```python
from build123d import *

# Parameters (mm, degrees)
F0_R     = 19.2
F1_DEPTH = 20
F2_R     = 2
F3_DEPTH = 25


with BuildPart() as f1:
    # F0 (on Top) → F1 (new body)
    with BuildSketch(Plane.XY):
        with BuildLine():
            ThreePointArc((14.459278, -13.962065), (18.636543, -7.529227), (20.1, 0))
            ThreePointArc((20.1, 0), (-7.529227, 18.636543), (-14.459278, -13.962065))
            ThreePointArc((-14.459278, -13.962065), (-7.854059, -18.501993), (0, -20.1))
            ThreePointArc((0, -20.1), (7.854059, -18.501993), (14.459278, -13.962065))
        make_face()
        Circle(F0_R, mode=Mode.SUBTRACT)
        Polygon((0, -23.1), (0, -20.1), (-20.239076, -20.1), (-30, -20.1), (-30, -23.1), align=None)
        with BuildLine():
            Line((20.239076, -20.1), (14.459278, -13.962065))
            ThreePointArc((14.459278, -13.962065), (7.854059, -18.501993), (0, -20.1))
            Line((0, -20.1), (20.239076, -20.1))
        make_face()
        with BuildLine():
            ThreePointArc((0, -20.1), (-7.854059, -18.501993), (-14.459278, -13.962065))
            Line((-14.459278, -13.962065), (-20.239076, -20.1))
            Line((-20.239076, -20.1), (0, -20.1))
        make_face()
        Polygon((20.239076, -20.1), (0, -20.1), (0, -23.1), (30, -23.1), (30, -20.1), align=None)
    extrude(amount=F1_DEPTH)

    # F2 (on face) → F3 (cut)
    with BuildSketch(Plane(origin=(0, -20.1, 0), x_dir=(-1, 0, 0), z_dir=(0, 1, 0))):
        with BuildLine():
            Line((-25.119538, 10.263338), (-25.119538, 8.263338))
            ThreePointArc((-25.119538, 8.263338), (-23.705324, 8.849124), (-23.119538, 10.263338))
            ThreePointArc((-23.119538, 10.263338), (-25.119538, 12.263338), (-27.119538, 10.263338))
            Line((-27.119538, 10.263338), (-25.119538, 10.263338))
        make_face()
        with BuildLine():
            ThreePointArc((-27.119538, 10.263338), (-26.533751, 8.849124), (-25.119538, 8.263338))
            Line((-25.119538, 8.263338), (-25.119538, 10.263338))
            Line((-25.119538, 10.263338), (-27.119538, 10.263338))
        make_face()
        with Locations((25.119538, 10.263338)):
            Circle(F2_R)
    extrude(amount=-F3_DEPTH, mode=Mode.SUBTRACT)


solid = f1.part
```
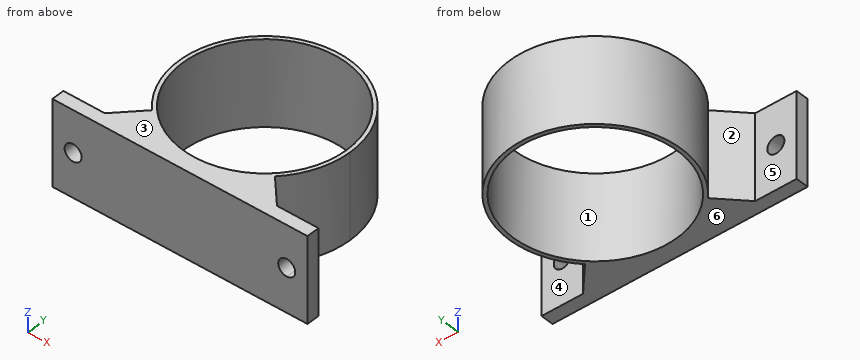
Could you check a few things on this model? Use its own coordinates, in mm. Face numbers are marked on the shaded views. A direction names the side the tool comes from. Round coordinates to 2 decimals unless told otherwise and drop trailing zeros. Loops run counter-clockwise (first coordinate to the right, second up) from the corner with the lowest first, then second, coordinate; pieces in that order, holes last. Notation, with made-up numbers: (52, -26.5) - (101, -26.5) arc R21 ccw to (101, -2.5) - close; hole circle Ø5 at (-10.75, -19.75). An arc over 180 degrees is marked (long way). Answer in a Markdown table with one row per item. Add a question column.
(1) For the marked faces 4, 5 and 6, which set-ups out of +Z, -Z, +X, -X, +Y, -Y let a thin tool reach every point of the face, with its end or its side?
(2) I'm going to push flat-ended pins straight in: pin 1 (3 mm diameter, centred on y = 12, z = 14, fed in from +X); pin 2 (6 mm diameter, centred on y = -14.5, z = 2.5, fed in from -X); pin 3 (8 mm diameter, centred on x = 26, z = 15, fed in from +Y). Where does each tip first touch, or does it pass through?
(3) I need wall thicknesses on line 1 along Y through (x, z) = (0, 7); line 2 along X through (y, z) = (-3, 15.25); line 3 along Y through (x, z) = (-24, 16.75). Which ranges of each line are inside material? Lowest first, please.
(4) If we section it at A-A (x = 0): Please give me the cut outline in (y, z), plus the area to 3 significant figures.
(5) If we section it at D-D (z = 9.5): Please give me the cut outline in (x, y).
(6) If we section it at B-B (z = 13.75): Please give me the cut outline in (x, y).
(7) If we section it at C-C (y = 16.5): Please give me the cut outline in (x, z), plus the area to 3 significant figures.
(8) If we mould it in two halves opening along X, with no side actions, what happens to the marked faces 1, 2 and 3? For each: pulls with the +X half, pulls with the -X half, needs draft (parallel to the pull), parting line crosses it, or undercut.
Model answer:
| question | item | result |
|---|---|---|
| 1 | face 4 | +Z, -Z, +X, +Y |
| 1 | face 5 | +Z, -Z, -X, +Y |
| 1 | face 6 | -Z, +X, -X, +Y, -Y |
| 2 | pin 1 | stops at x = 17.14 |
| 2 | pin 2 | stops at x = -17.79 |
| 2 | pin 3 | stops at y = -20.1 |
| 3 | line 1 | y = -23.1 to -19.2, 19.2 to 20.1 |
| 3 | line 2 | x = -19.87 to -18.96, 18.96 to 19.87 |
| 3 | line 3 | y = -23.1 to -20.1 |
| 4 | outline | (-23.1, 0) - (-19.2, 0) - (-19.2, 20) - (-23.1, 20) - close; (19.2, 0) - (20.1, 0) - (20.1, 20) - (19.2, 20) - close |
| 4 | area | 96.0 mm² |
| 5 | outline | (-30, -23.1) - (-26.97, -23.1) - (-26.97, -20.1) - (-30, -20.1) - close; (-23.27, -23.1) - (23.27, -23.1) - (23.27, -20.1) - (20.24, -20.1) - (14.46, -13.96) arc R20.1 ccw to (20.1, 0) arc R20.1 ccw (long way) to (-14.46, -13.96) - (-20.24, -20.1) - (-23.27, -20.1) - close; (26.97, -23.1) - (30, -23.1) - (30, -20.1) - (26.97, -20.1) - close; hole circle Ø38.4 at (0, 0) |
| 6 | outline | (-30, -23.1) - (30, -23.1) - (30, -20.1) - (20.24, -20.1) - (14.46, -13.96) arc R20.1 ccw to (20.1, 0) arc R20.1 ccw (long way) to (-14.46, -13.96) - (-20.24, -20.1) - (-30, -20.1) - close; hole circle Ø38.4 at (0, 0) |
| 7 | outline | (-11.48, 0) - (-9.82, 0) - (-9.82, 20) - (-11.48, 20) - close; (9.82, 0) - (11.48, 0) - (11.48, 20) - (9.82, 20) - close |
| 7 | area | 66.4 mm² |
| 8 | face 1 | undercut |
| 8 | face 2 | pulls with the -X half |
| 8 | face 3 | needs draft |
